```python
from build123d import *

# Parameters (mm, degrees)
SKETCH_1_W              = 120
SKETCH_1_H              = 40
EXTRUDE_1_DEPTH         = 15
SKETCH_5_R              = 6
CUT_EXTRUDE_2_DEPTH     = 20
M18X1_5_1_D             = 16.5
SKETCH_8_W              = 45
SKETCH_8_H              = 16
CUT_EXTRUDE_3_DEPTH     = 31
FILLET_1_R              = 10
HOLE_WIZARD_M12_1_D     = 10.2
HOLE_WIZARD_M12_1_DEPTH = 15
HOLE_WIZARD_M12_1_TIP   = 3.064389157


with BuildPart() as part:
    # 草图1 → 凸台-拉伸1 (new body, symmetric)
    with BuildSketch(Plane.XY):
        Rectangle(SKETCH_1_W, SKETCH_1_H)
    extrude(amount=EXTRUDE_1_DEPTH, both=True)

    # 草图5 → 切除-拉伸2 (cut)
    with BuildSketch(Plane(origin=(0, -20, 0), x_dir=(-1, 0, 0), z_dir=(0, -1, 0))):
        with Locations((45, 0)):
            Circle(SKETCH_5_R)
        with Locations((-45, 0)):
            Circle(SKETCH_5_R)
    extrude(amount=-CUT_EXTRUDE_2_DEPTH, mode=Mode.SUBTRACT)

    # M18x1.5 螺纹孔1 (through all)
    with Locations(Plane.XY.offset(15)):
        with Locations((0, 0)):
            Hole(M18X1_5_1_D / 2)

    # 草图8 → 切除-拉伸3 (cut, through all)
    with BuildSketch(Plane.XY.offset(15)):
        with Locations((-37.5, 0)):
            Rectangle(SKETCH_8_W, SKETCH_8_H)
        with Locations((37.5, 0)):
            Rectangle(SKETCH_8_W, SKETCH_8_H)
    extrude(amount=-CUT_EXTRUDE_3_DEPTH, mode=Mode.SUBTRACT)

    # 圆角1
    fillet_1_edges = [part.edges().sort_by_distance(p)[0] for p in [
        (-60, 14, 15),
        (-60, -14, -15),
        (-60, -14, 15),
        (60, -14, 15),
        (60, 14, -15),
        (60, 14, 15),
        (-60, 14, -15),
        (60, -14, -15),
    ]]
    fillet(fillet_1_edges, radius=FILLET_1_R)

    # M12 螺纹孔1
    with Locations(Plane(origin=(0, 20, 0), x_dir=(1, 0, 0), z_dir=(0, 1, 0))):
        with Locations((-45, 0), (45, 0)):
            Hole(HOLE_WIZARD_M12_1_D / 2, depth=HOLE_WIZARD_M12_1_DEPTH)
            with Locations((0, 0, -(HOLE_WIZARD_M12_1_DEPTH + HOLE_WIZARD_M12_1_TIP / 2))):  # 118° drill point
                Cone(0, HOLE_WIZARD_M12_1_D / 2, HOLE_WIZARD_M12_1_TIP, mode=Mode.SUBTRACT)


solid = part.part
```
Can you work these out from the model? Positions are in its coordinate system, mm. A direction names the side the tool comes from. Coordinates: 2 decimals unless noted, no trailing zeros. Loops run counter-clockwise (first coordinate to the right, second up) from the corner with the lowest first, then second, coordinate; pieces in that order, holes last.
1) Which directions (+Z, -Z, +X, -X, +Y, -Y) give clear straight access to the entire face, cutting with the end or side of a thin tool? Please do faces 1 (the cylindrical face through (-39, -14, 0)), 2 (the flat face through (-15, 0, 0)), 3 (the flat face through (37, -8, 0)).
2) Thinking about a two-plate mould opening in X: for faces 4 (the cylindrical face through (-7.62, -3.16, -0.21)), 5 (the cylindrical face through (56.99, -13.92, -12.15)), 6 (the flat face through (-60, -14, 0)), which applies, pulls with the +X half, pulls with the -X half, needs draft (parallel to the pull), parting line crosses it, or undercut?
3) Imagine slicing it at A-A on z = 0. State how many separate pieces and enclosed holes the cut face has, plus the area to 3 significant figures.
4) Imagine slicing it at C-C on y = 0. List the corners of the cut face in (x, z) for me.
5) Imagine slicing it at D-D on x = -45. List the corners of the cut face in (y, z) for me.
6) I need wall thicknesses on probe 1 along X at (y, z) = (-12.25, 0); probe 2 along Z at (x, y) = (-45, -11); probe 3 along Y at (x, z) = (43, 9). Which ranges of each line are inside material? Lowest first, please.
7) Imagine slicing it at B-B on x = 0. List the corners of the cut face in (y, z) for me, plus the area to 3 significant figures.
8) For pin 1 (5 mm diameter, centred on y = 0.5, z = 7.5, fed in from -X); pin 2 (7 mm diameter, centred on x = 45, z = 0, fed in from -Y), each with a flat end and sliding along its axis, tell me the tip position at first contact or that it passes through.
Completed:
1. face 1: -Y
1. face 2: +Z, -Z, -X
1. face 3: +Z, -Z, +X
2. face 4: undercut
2. face 5: pulls with the +X half
2. face 6: pulls with the -X half
3. separate pieces: 5
3. enclosed holes: 1
3. area: 2,610 mm2
4. outline: (-15, -15) - (-8.25, -15) - (-8.25, 15) - (-15, 15) - close; (8.25, -15) - (15, -15) - (15, 15) - (8.25, 15) - close
5. outline: (-20, -15) - (-8, -15) - (-8, -6) - (-20, -6) - close; (-20, 6) - (-8, 6) - (-8, 15) - (-20, 15) - close; (8, -15) - (20, -15) - (20, -5.1) - (8, -5.1) - close; (8, 5.1) - (20, 5.1) - (20, 15) - (8, 15) - close
6. probe 1: x = -60 to -51, -39 to 39, 51 to 60
6. probe 2: z = -15 to -6, 6 to 15
6. probe 3: y = -20 to -8, 8 to 20
7. outline: (-20, -15) - (-8.25, -15) - (-8.25, 15) - (-20, 15) - close; (8.25, -15) - (20, -15) - (20, 15) - (8.25, 15) - close
7. area: 705 mm2
8. pin 1: stops at x = -15
8. pin 2: passes through
